Here's how the part is built. I have some questions about the finished solid (model axes, mm). Face numbers are marked on the shaded views. A direction names the side the tool comes from. Coordinates: 2 decimals unless noted, no trailing zeros. Loops run counter-clockwise (first coordinate to the right, second up) from the corner with the lowest first, then second, coordinate; pieces in that order, holes last. Notation, with made-up numbers: (-12, 72.5) -> (5, 72.5) arc R22 ccw to (5, 91.5) -> close; hole circle Ø3 at (80, 59.5). An arc over 180 degrees is marked (long way). Answer as a JSON object with one key per item and string values. Group by question number.
Q1. I'm going to push a flat-ended pin straight in: pin 1 (1 mm diameter, centred on x = 6.5, y = -6, fed in from +Z). Where does the tip first touch, or does it pass through?
Q2. Thinking about a two-plate mould opening in Y: for the marked faces 1, 2 and 3, which applies, released by +Y, released by -Y, zero draft, split by the parting line, or undercut?
Q3. I want a section at A-A on y = 0. Write out the boundary of the cut face in (x, z), then the cut area to 3 significant figures.
Q4. I need wall thicknesses on line 1 (Y direction, x = 0, z = 2.3); line 2 (Z direction, x = -5.5, y = -6.75); line 3 (Z direction, x = -5.5, y = -1). Which ranges of each line are inside material? Lowest first, please.
Q5. I want a section at D-D on y = 8.25. Write out the boundary of the cut face in (x, z), then the cut area to 3 significant figures.
Q6. On a 3-axis mill with a long thin cutter (end or side, diameter ignored), from which of +Z, -Z, +X, -X, +Y, -Y can I reach the whole of each face in a straight line? I mean the marked faces 4 and 5. Say none if no direction works.
Q7. I want a section at C-C on z = 1.5. Write out the boundary of the cut face in (x, y), then the cut area to 3 significant figures.
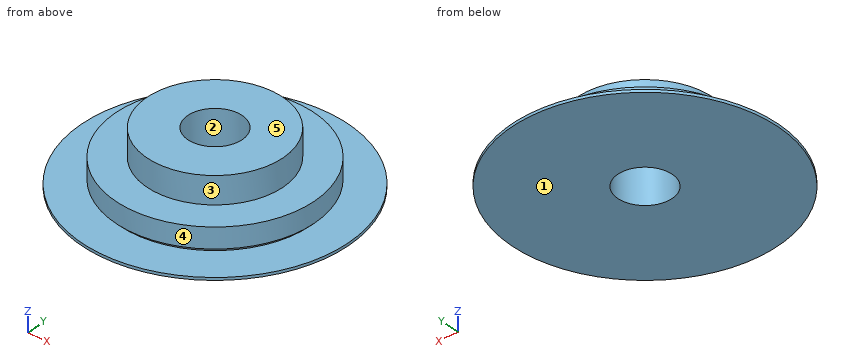
```python
from build123d import *

# Parameters (mm, degrees)
F0_R     = 7.3
F1_DEPTH = 2
F2_R     = 5
F3_DEPTH = 2
F4_SIZE  = 0.5
F5_R     = 2
F6_DEPTH = 4.001
F7_R     = 9.8
F7_R_2   = 6.8
F8_DEPTH = 0.2


with BuildPart() as f1:
    # F0 (on Top) → F1 (new body)
    with BuildSketch(Plane.XY):
        Circle(F0_R)
    extrude(amount=F1_DEPTH)

    # F2 (on face) → F3 (join)
    with BuildSketch(Plane.XY.offset(2)):
        Circle(F2_R)
    extrude(amount=F3_DEPTH)

    # F4
    f4_edges = [f1.edges().sort_by_distance(p)[0] for p in [
        (-7.3, 0, 0),
    ]]
    chamfer(f4_edges, length=F4_SIZE)

    # F5 (on face) → F6 (cut, through all)
    with BuildSketch(Plane(origin=(0, 0, 0), x_dir=(1, 0, 0), z_dir=(0, 0, -1))):
        Circle(F5_R)
    extrude(amount=-F6_DEPTH, mode=Mode.SUBTRACT)

    # F7 (on face) → F8 (join)
    with BuildSketch(Plane(origin=(0, 0, 0), x_dir=(1, 0, 0), z_dir=(0, 0, -1))):
        Circle(F7_R)
        Circle(F7_R_2, mode=Mode.SUBTRACT)
    extrude(amount=-F8_DEPTH)


solid = f1.part
```
Result set:
{
 "1": {"pin 1": "stops at z = 0.2"},
 "2": {"face 1": "zero draft", "face 2": "undercut", "face 3": "split by the parting line"},
 "3": {"outline": "(-9.8, 0) -> (-2, 0) -> (-2, 4) -> (-5, 4) -> (-5, 2) -> (-7.3, 2) -> (-7.3, 0.5) -> (-7, 0.2) -> (-9.8, 0.2) -> close; (2, 0) -> (9.8, 0) -> (9.8, 0.2) -> (7, 0.2) -> (7.3, 0.5) -> (7.3, 2) -> (5, 2) -> (5, 4) -> (2, 4) -> close", "area": "34.1 mm²"},
 "4": {"line 1": "y = -5 to -2, 2 to 5", "line 2": "z = 0 to 0.2", "line 3": "z = 0 to 2"},
 "5": {"outline": "(-5.29, 0) -> (5.29, 0) -> (5.29, 0.2) -> (-5.29, 0.2) -> close", "area": "2.12 mm²"},
 "6": {"face 4": "+Z", "face 5": "+Z, +X, -X, +Y, -Y"},
 "7": {"outline": "circle Ø14.6 at (0, 0); hole circle Ø4 at (0, 0)", "area": "155 mm²"}
}
